Geometry: see drawing. Coordinates: mm, zero at the bounding-box minimum. Give positions to 0.01 mm unless a question says otherwise; leave off trailing zeros. Write each loop counter-clockwise with the first axis right and the second up, starting at its lowest first coordinate (ties: lowest second). Pieces come first, ordered by that corner, then holes. Notation, with made-up numbers: M 11.25,-25.5 L 23.25,-25.5 A8 cw 23.25,-13.5 Z; hole C -24.5,48.25 d1. An arc over 180 degrees is marked long. Use a Markdown table: item, result. Add a question column.
1) Line query: line 1 (Y direction, x = 2.75, z = 8.25); line 2 (X direction, y = 8, z = 4.5); line 3 (Z direction, x = 3.75, y = 3) (1 decimal). Output: solid intervals per line, ascending.
2) Pin query (flat end, axial travel): pin 1 (6 mm diameter, centred on y = 53.5, z = 5.5, fed in from -X); pin 2 (3 mm diameter, centred on y = 19, z = 3.5, fed in from +X); pin 3 (8 mm diameter, centred on x = 6, y = 36.5, fed in from +Z). Return the tip coordinate at first contact, or that it passes through.
3) Draft query along Z for the marked faces 1, 2, 3 and 4. Return one class per face: +Z half, -Z half, draft (parallel to the pull), parting line (faces both ways), or undercut.
4) Section A-A on y = 61.5. Return the cut outline in (x, z) (1 decimal).
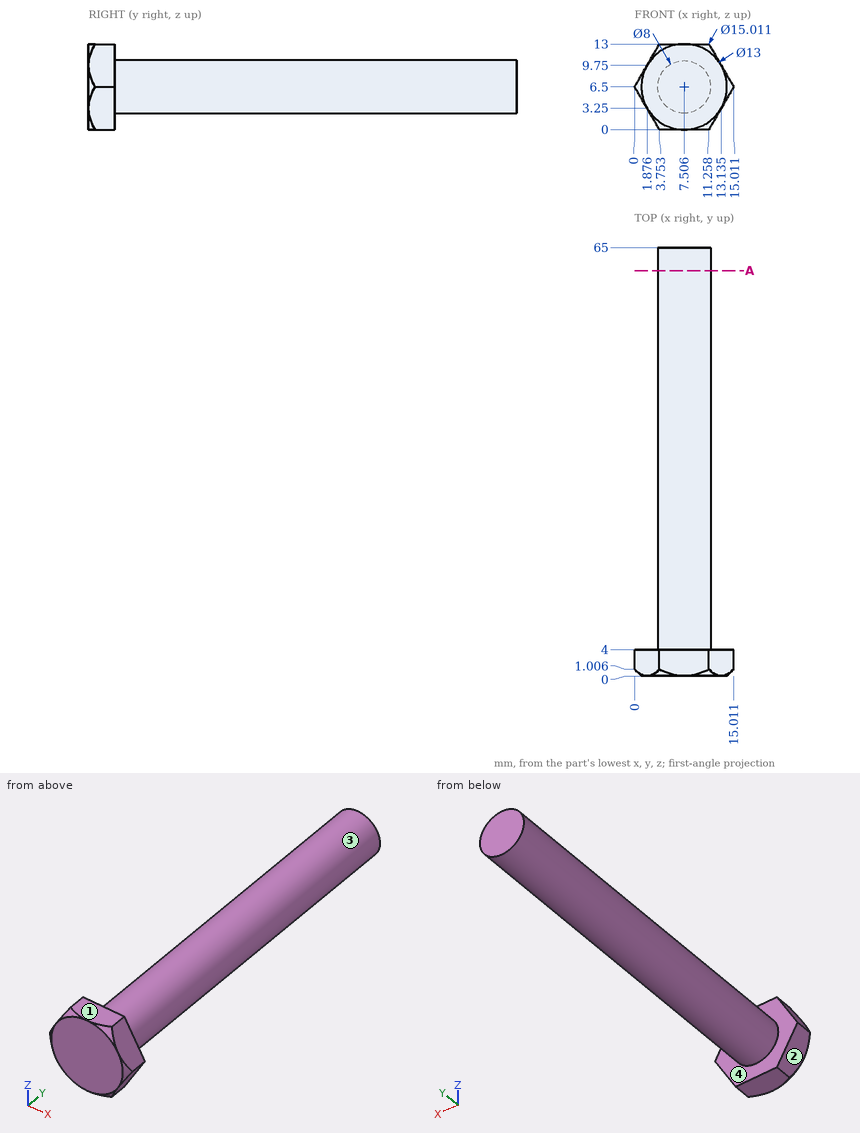
Found:
| question | item | result |
|---|---|---|
| 1 | line 1 | 0 to 4 |
| 1 | line 2 | 4.04 to 10.97 |
| 1 | line 3 | 0 to 13 |
| 2 | pin 1 | x = 3.51 |
| 2 | pin 2 | x = 11.21 |
| 2 | pin 3 | z = 10.5 |
| 3 | face 1 | +Z half |
| 3 | face 2 | -Z half |
| 3 | face 3 | parting line |
| 3 | face 4 | draft |
| 4 | outline | C 7.5,6.5 d8 |
